Job drawing, mm, ordinate dimensions from the low corner. One solid piece. A direction names the side the tool comes from. Give positions to 0.01 mm unless a question says otherwise; leave off trailing zeros. Write each loop counter-clockwise with the first axis right and the second up, starting at its lowest first coordinate (ties: lowest second). Pieces come first, ordered by that corner, then holes. Notation, with made-up numbers: (5.25, -33) - (17.25, -33) arc R13 ccw to (17.25, -9) - close; hole circle Ø8 at (-24, 21.25). An arc over 180 degrees is marked (long way). Use a Markdown table: item, result. Add a question column.
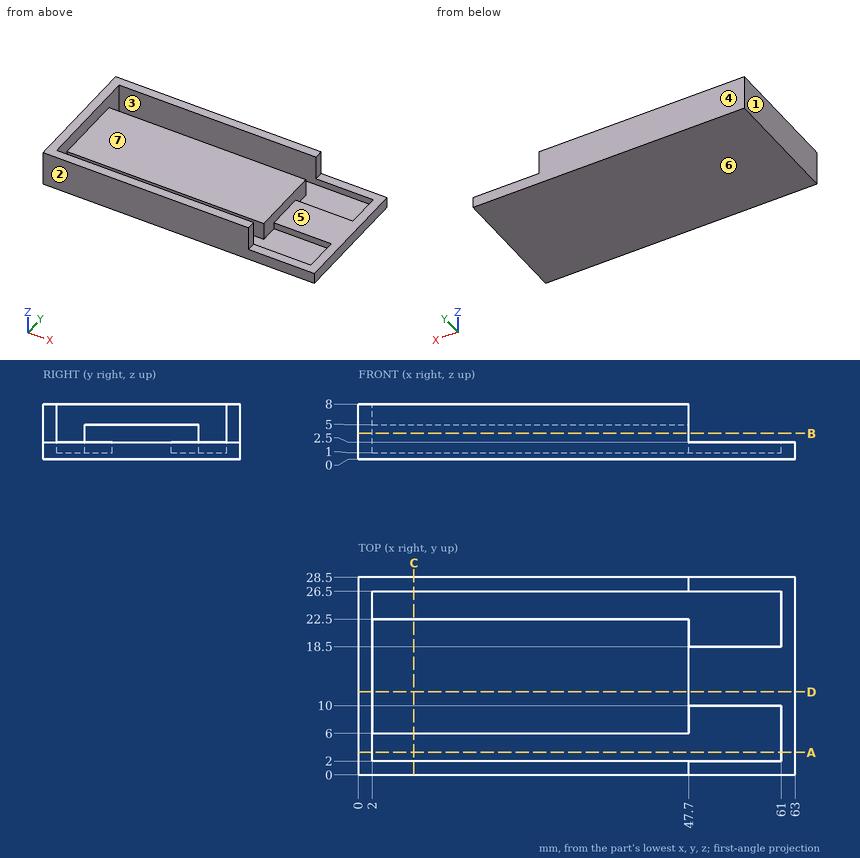
(1) Band-saw the part on B-B (z = 3.75). Write the cut outline in (x, y), then the cut area to 3 significant figures.
(2) Which spindle directions (+Z, -Z, +X, -X, +Y, -Y) get a long thin tool onto all of the face, cutting with end or side? Do the marked faces 5, 6 and 7. Say none if no direction does.
(3) Band-saw the part on D-D (y = 12). Write the cut outline in (x, z), then the cut area to 3 significant figures.
(4) Band-saw the part on C-C (x = 8). Write the cut outline in (y, z).
(5) Probe probe 1 along Y at (x, z) = (18.5, 3.75); probe 2 along Y at (x, z) = (49.5, 1.5); probe 3 along X at (y, z) = (5.25, 1.5). List the from-to ranges inside material, lowest first. Write a range as [from, to].
(6) Band-saw the part on A-A (y = 3.25). Write the cut outline in (x, z).
(7) Two-plate mould, pull along Y, no slides. Class the marked faces 1, 2, 3 and 4: +Y half, -Y half, draft (parallel to the pull), parting line (faces both ways), or undercut.
(8) Flat gauge pins, fed straight in: pin 1 (2 mm diameter, centred on y = 0.5, z = 4, fed in from +X); pin 2 (6.5 mm diameter, centred on x = 19.5, y = 4.5, fed in from +Z); pin 3 (13 mm diameter, centred on x = 22, y = 17.5, fed in from +Z); pin 4 (7.5 mm diameter, centred on x = 57, y = 15, fed in from +Z). Where does each tip first touch, or does it go through?
Model answer:
| question | item | result |
|---|---|---|
| 1 | outline | (0, 0) - (47.7, 0) - (47.7, 2) - (2, 2) - (2, 6) - (47.7, 6) - (47.7, 22.5) - (2, 22.5) - (2, 26.5) - (47.7, 26.5) - (47.7, 28.5) - (0, 28.5) - close |
| 1 | area | 994 mm^2 |
| 2 | face 5 | +Z, +X, +Y, -Y |
| 2 | face 6 | -Z, +X, -X, +Y, -Y |
| 2 | face 7 | +Z, +X |
| 3 | outline | (0, 0) - (63, 0) - (63, 2.5) - (47.7, 2.5) - (47.7, 5) - (2, 5) - (2, 8) - (0, 8) - close |
| 3 | area | 283 mm^2 |
| 4 | outline | (0, 0) - (28.5, 0) - (28.5, 8) - (26.5, 8) - (26.5, 1) - (22.5, 1) - (22.5, 5) - (6, 5) - (6, 1) - (2, 1) - (2, 8) - (0, 8) - close |
| 5 | probe 1 | y = [0, 2], [6, 22.5], [26.5, 28.5] |
| 5 | probe 2 | y = [0, 2], [10, 18.5], [26.5, 28.5] |
| 5 | probe 3 | x = [0, 2], [61, 63] |
| 6 | outline | (0, 0) - (63, 0) - (63, 2.5) - (61, 2.5) - (61, 1) - (2, 1) - (2, 8) - (0, 8) - close |
| 7 | face 1 | draft |
| 7 | face 2 | -Y half |
| 7 | face 3 | undercut |
| 7 | face 4 | +Y half |
| 8 | pin 1 | stops at x = 47.7 |
| 8 | pin 2 | stops at z = 8 |
| 8 | pin 3 | stops at z = 5 |
| 8 | pin 4 | stops at z = 2.5 |
